Geometry: final body of the model. Coordinates: model frame, mm. A direction names the side the tool comes from. Round coordinates to 2 decimals unless told otherwise and drop trailing zeros. Order: outer loops, then holes, each group sorted by start corner. A loop starts at its lowest first (then second) coordinate and runs counter-clockwise, first axis right, second up. Notation, with made-up numbers: (5, 73.5) - (45, 73.5) arc R19 ccw to (45, 82.5) - close; hole circle Ø10 at (5, 63). An arc over 180 degrees is marked (long way). Put each result on its own line as item: value. Start each with the question number.
(1) Section C-C (z = 1). Output: boundary loops of the cut face in (x, y), and give its area (3 significant figures).
(2) Pin query (flat end, axial travel): P1, Ø8, axis at x = 18, z = -7.5, coming from the +Y side; P2, Ø0.5, axis at x = 34, y = -4, coming from the -Z side; P3, Ø1, axis at x = -25.5, y = 9.5, coming from the +Z side; P4, Ø2.5, axis at x = -7.5, z = -1.5, coming from the +Y side. Return the tip coordinate at first contact, or that it passes through.
(3) Pull-direction query (X, two-part tool) for faces 4 (the face through (27, 24.5, -5)), 5 (the face through (0, 0, -3)), 6 (the face through (-27.5, 0, -8)); classes: released by +X, released by -X, zero draft, split by the parting line, or undercut.
(4) Section A-A (x = 7). Output: boundary loops of the cut face in (y, z).
(5) Access query for faces 1 (the face through (19.5, 17, -1)), 2 (the face through (27, -24.5, -5)), 3 (the face through (-29.5, 0, -8)). Directions: +Z, -Z, +X, -X, +Y, -Y. A direction counts if a zero-diameter tool reaches every point of the face in a straight line with its end or side. Return the directions, or none.
(6) Section D-D (x = -9.5). Output: boundary loops of the cut face in (y, z).
(7) Material intervals for L1, parallel to Z at x = -30, y = -16; L2, parallel to X at y = 20, z = -1.5; L3, parallel to Z at x = -25, y = -15.5, sorted ascending. Write a range as [from, to].
(8) Section B-B (z = -9). Count the separate pieces of the cut face and the enclosed holes in it, and give its area (3 significant figures).
Autodesk Inventor part; units mm, degrees
ref_plane "YZ Plane" through (0, 0, 0) normal (1, 0, 0) x (0, 1, 0)
ref_plane "XZ Plane" through (0, 0, 0) normal (0, 1, 0) x (-1, 0, 0)
ref_plane "XY Plane" through (0, 0, 0) normal (0, 0, 1) x (1, 0, 0)
sketch "Sketch2" plane through (0, 0, 0) normal (0, 0, 1) x (1, 0, 0)
  line L0 (-8.5, 4.5) -> (8.5, 4.5)
  line L1 (8.5, 4.5) -> (8.5, -4.5)
  line L2 (8.5, -4.5) -> (-8.5, -4.5)
  line L3 (-8.5, -4.5) -> (-8.5, 4.5)
  line L4 (8.5, 4.5) -> (-8.5, -4.5) construction
  line L5 (8.5, -4.5) -> (-8.5, 4.5) construction
  point P0 (0, 0)
  dimension "d12" = 17
  dimension "d13" = 9
extrude "Extrusion2" add sketch "Sketch2" along normal blind 3
sketch "Sketch3" plane through (0, 0, 0) normal (0, 0, -1) x (-1, 0, 0)
  line L0 (-19.5, 9.5) -> (19.5, 9.5)
  line L1 (19.5, 9.5) -> (19.5, -9.5)
  line L2 (19.5, -9.5) -> (-19.5, -9.5)
  line L3 (-19.5, -9.5) -> (-19.5, 9.5)
  line L4 (-19.5, 9.5) -> (19.5, -9.5) construction
  line L5 (19.5, 9.5) -> (-19.5, -9.5) construction
  line L6 (8.5, 4.5) -> (-8.5, 4.5)
  line L7 (-8.5, 4.5) -> (-8.5, -4.5)
  line L8 (19.5, 15) -> (-19.5, 15) construction
  line L9 (-19.5, 15) -> (-19.5, -15) construction
  line L10 (-19.5, -15) -> (19.5, -15) construction
  line L11 (19.5, -15) -> (19.5, 15) construction
  line L12 (19.5, -15) -> (-19.5, 15) construction
  line L13 (-19.5, -15) -> (19.5, 15) construction
  line L14 (-19.5, 24.5) -> (-39.5, 24.5)
  line L15 (-19.5, 9.5) -> (-19.5, 24.5)
  line L16 (-39.5, 24.5) -> (-39.5, 0)
  line L17 (0, 0) -> (15.34, 0) construction
  line L18 (-19.5, -24.5) -> (-39.5, -24.5)
  line L19 (-19.5, -9.5) -> (-19.5, -24.5)
  line L20 (-39.5, -24.5) -> (-39.5, 0)
  line L21 (0, 0) -> (0, 17) construction
  line L22 (19.5, 24.5) -> (39.5, 24.5)
  line L23 (19.5, 9.5) -> (19.5, 24.5)
  line L24 (39.5, 24.5) -> (39.5, 0)
  line L25 (19.5, -9.5) -> (19.5, -24.5)
  line L26 (19.5, -24.5) -> (39.5, -24.5)
  line L27 (39.5, -24.5) -> (39.5, 0)
  dimension "d16" = 11
  dimension "d17" = 5
  dimension "d18" = 39
  dimension "d39" = 19
  dimension "d55" = 39
  dimension "d56" = 30
  dimension "d57" = 15
  dimension "d58" = 20
  dimension "d78" = 49
extrude "Extrusion3" add sketch "Sketch3" along normal blind 3
sketch "Sketch6" plane through (-19.5, 9.5, 0) normal (0, 1, 0) x (1, 0, 0)
  point P0 (19.5, 0)
sketch "Sketch7" plane through (19.5, 24.5, 0) normal (0, 1, 0) x (1, 0, 0)
  line L0 (20, 3) -> (20, 13)
  line L1 (20, 13) -> (19, 13)
  line L2 (19, 13) -> (19, 3)
  line L3 (-19.5, 0) -> (-19.5, 8) construction
  line L4 (20, 3) -> (19, 3)
  line L5 (18, 3) -> (18, 13)
  line L6 (18, 13) -> (17, 13)
  line L7 (17, 13) -> (17, 3)
  line L8 (18, 3) -> (17, 3)
  line L9 (16, 3) -> (16, 13)
  line L10 (16, 13) -> (15, 13)
  line L11 (15, 13) -> (15, 3)
  line L12 (16, 3) -> (15, 3)
  line L13 (14, 3) -> (14, 13)
  line L14 (14, 13) -> (13, 13)
  line L15 (13, 13) -> (13, 3)
  line L16 (14, 3) -> (13, 3)
  line L17 (12, 3) -> (12, 13)
  line L18 (12, 13) -> (11, 13)
  line L19 (11, 13) -> (11, 3)
  line L20 (12, 3) -> (11, 3)
  line L21 (10, 3) -> (10, 13)
  line L22 (10, 13) -> (9, 13)
  line L23 (9, 13) -> (9, 3)
  line L24 (10, 3) -> (9, 3)
  line L25 (8, 3) -> (8, 13)
  line L26 (8, 13) -> (7, 13)
  line L27 (7, 13) -> (7, 3)
  line L28 (8, 3) -> (7, 3)
  line L29 (6, 3) -> (6, 13)
  line L30 (6, 13) -> (5, 13)
  line L31 (5, 13) -> (5, 3)
  line L32 (6, 3) -> (5, 3)
  line L33 (4, 3) -> (4, 13)
  line L34 (4, 13) -> (3, 13)
  line L35 (3, 13) -> (3, 3)
  line L36 (4, 3) -> (3, 3)
  line L37 (0, 0) -> (-39, 0)
  line L38 (-59, 3) -> (-59, 13)
  line L39 (-59, 13) -> (-58, 13)
  line L40 (-58, 13) -> (-58, 3)
  line L41 (-59, 3) -> (-58, 3)
  line L42 (-57, 3) -> (-57, 13)
  line L43 (-57, 13) -> (-56, 13)
  line L44 (-56, 13) -> (-56, 3)
  line L45 (-57, 3) -> (-56, 3)
  line L46 (-55, 3) -> (-55, 13)
  line L47 (-55, 13) -> (-54, 13)
  line L48 (-54, 13) -> (-54, 3)
  line L49 (-55, 3) -> (-54, 3)
  line L50 (-53, 3) -> (-53, 13)
  line L51 (-53, 13) -> (-52, 13)
  line L52 (-52, 13) -> (-52, 3)
  line L53 (-53, 3) -> (-52, 3)
  line L54 (-51, 3) -> (-51, 13)
  line L55 (-51, 13) -> (-50, 13)
  line L56 (-50, 13) -> (-50, 3)
  line L57 (-51, 3) -> (-50, 3)
  line L58 (-49, 3) -> (-49, 13)
  line L59 (-49, 13) -> (-48, 13)
  line L60 (-48, 13) -> (-48, 3)
  line L61 (-49, 3) -> (-48, 3)
  line L62 (-47, 3) -> (-47, 13)
  line L63 (-47, 13) -> (-46, 13)
  line L64 (-46, 13) -> (-46, 3)
  line L65 (-47, 3) -> (-46, 3)
  line L66 (-45, 3) -> (-45, 13)
  line L67 (-45, 13) -> (-44, 13)
  line L68 (-44, 13) -> (-44, 3)
  line L69 (-45, 3) -> (-44, 3)
  line L70 (-43, 3) -> (-43, 13)
  line L71 (-43, 13) -> (-42, 13)
  line L72 (-42, 13) -> (-42, 3)
  line L73 (-43, 3) -> (-42, 3)
  dimension "d59" = 10
  dimension "d60" = 1
  dimension "d71" = 2
  dimension "d76" = 79
  dimension "d77" = 3
extrude "Extrusion6" add sketch "Sketch7" against normal blind 49
properties part number "SensorCooler01"
Checks:
1. outline: (-8.5, -4.5) - (8.5, -4.5) - (8.5, 4.5) - (-8.5, 4.5) - close
1. area: 153 mm²
2. P1: passes through
2. P2: stops at z = -3
2. P3: stops at z = 0
2. P4: stops at y = 9.5
3. face 4: zero draft
3. face 5: undercut
3. face 6: undercut
4. outline: (-9.5, -3) - (9.5, -3) - (9.5, 0) - (4.5, 0) - (4.5, 3) - (-4.5, 3) - (-4.5, 0) - (-9.5, 0) - close
5. face 1: +Z, -Z, +Y
5. face 2: +Z, -Z, +X, -X, -Y
5. face 3: -Z, +Y, -Y
6. outline: (-9.5, -3) - (9.5, -3) - (9.5, 0) - (-9.5, 0) - close
7. L1: z = [-3, 0]
7. L2: x = [-39.5, -19.5], [19.5, 39.5]
7. L3: z = [-13, 0]
8. separate pieces: 18
8. enclosed holes: 0
8. area: 882 mm²
